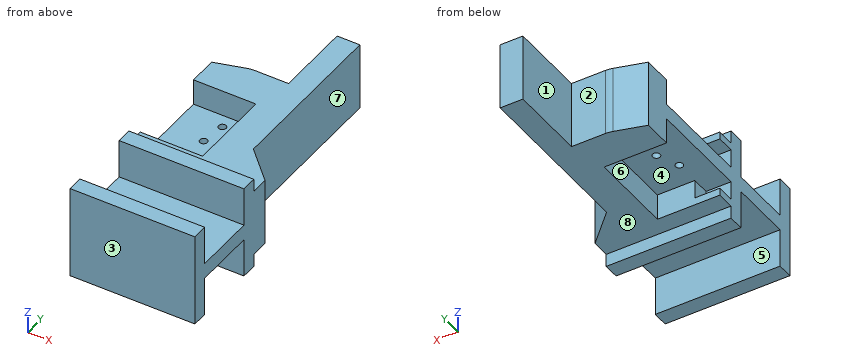
Autodesk Inventor part; units mm, degrees
ref_plane "YZ Plane" through (0, 0, 0) normal (1, 0, 0) x (0, 1, 0)
ref_plane "XZ Plane" through (0, 0, 0) normal (0, 1, 0) x (-1, 0, 0)
ref_plane "XY Plane" through (0, 0, 0) normal (0, 0, 1) x (1, 0, 0)
sketch "Sketch1" plane through (0, 0, 0) normal (0, 0, 1) x (1, 0, 0)
  line L0 (-9.525, 0) -> (9.525, 0)
  line L1 (9.525, 0) -> (9.525, 44.45)
  line L2 (9.525, 44.45) -> (5.715, 44.45)
  line L3 (5.715, 44.45) -> (4.891, 28.7274)
  line L4 (4.891, 28.7274) -> (-9.525, 28.7274)
  line L5 (-9.525, 28.7274) -> (-9.525, 0)
  point P0 (0, 0)
  point P1 (0, 0)
  dimension "d0" = 44.45
  dimension "d1" = 15.24
  dimension "d2" = 15.7226
  dimension "d3" = 19.05
  dimension "d14" = 93
extrude "Extrusion1" add sketch "Sketch1" along normal mid plane 15.7226
sketch "Sketch2" plane through (0, 0, 0) normal (1, 0, 0) x (0, 1, 0)
  line L0 (-19.05, 9.525) -> (-19.05, -9.525)
  line L1 (-19.05, -9.525) -> (-15.875, -9.525)
  line L2 (-15.875, -9.525) -> (-15.875, -1.5875)
  line L3 (-15.875, -1.5875) -> (-3.175, -1.5875)
  line L4 (-3.175, -1.5875) -> (-3.175, -9.525)
  line L5 (-3.175, -9.525) -> (0, -9.525)
  line L6 (0, -9.525) -> (0, 9.525)
  line L7 (0, 9.525) -> (-3.175, 9.525)
  line L8 (-3.175, 9.525) -> (-3.175, 1.5875)
  line L9 (-3.175, 1.5875) -> (-15.875, 1.5875)
  line L10 (-15.875, 1.5875) -> (-15.875, 9.525)
  line L11 (-15.875, 9.525) -> (-19.05, 9.525)
  line L12 (0, -7.8613) -> (0, 7.8613)
  point P0 (0, 0)
  point P1 (0, 0)
  dimension "d6" = 19.05
  dimension "d7" = 19.05
  dimension "d8" = 3.175
  dimension "d9" = 3.175
extrude "Extrusion2" add sketch "Sketch2" along normal mid plane 19.05
sketch "Sketch6" plane through (0, 0, 7.8613) normal (0, 0, 1) x (1, 0, 0)
  line L0 (4.891, 28.7274) -> (9.525, 28.7274)
  line L1 (9.525, 28.7274) -> (9.525, 44.45)
  line L2 (9.525, 44.45) -> (4.891, 44.45)
  line L3 (4.891, 44.45) -> (4.891, 28.7274)
  point P0 (0, 0)
extrude "Extrusion3" add sketch "Sketch6" against normal blind 15.7226
sketch "Sketch9" plane through (0, 0, 7.8613) normal (0, 0, 1) x (1, 0, 0)
  line L0 (4.891, 44.45) -> (4.891, 28.7274)
  line L1 (-9.525, 28.7274) -> (-9.525, 0)
  line L2 (4.891, 28.7274) -> (-2.729, 28.7274)
  line L3 (4.891, 28.7274) -> (-9.525, 28.7274)
  line L4 (-9.525, 28.7274) -> (-9.525, 26.7462)
  line L5 (-9.525, 26.7462) -> (-2.729, 28.7274)
  point P0 (0, 0)
  dimension "d22" = 14.416
  dimension "d23" = 7.62
  dimension "d24" = 1.9812
extrude "Extrusion5" cut sketch "Sketch9" against normal blind 25.4
fillet "Fillet2" radius 5.08 1 edges at (-2.729, 28.7274, 0)
sketch "Sketch10" plane through (-9.525, -15.875, 1.5875) normal (0, 0, 1) x (1, 0, 0)
  circle A0 centre (9.525, 6.35) radius 0.635
  line L0 (0, 0) -> (0, 12.7)
  line L1 (19.05, -3.175) -> (0, -3.175)
  point P0 (9.525, 15.875)
  dimension "d28" = 9.525
  dimension "d29" = 9.525
  dimension "d30" = 1.27
extrude "Extrusion6" cut sketch "Sketch10" against normal blind 25.4
sketch "Sketch12" plane through (-9.525, -15.875, -1.5875) normal (-1, 0, 0) x (0, 0, 1)
  line L0 (-6.2738, 60.325) -> (-6.2738, 15.875)
  line L1 (9.4488, 42.6212) -> (9.4488, 15.875)
  line L2 (-6.2738, 36.7601) -> (9.4488, 36.7601)
  line L3 (9.4488, 36.7601) -> (9.4488, 19.5053)
  line L4 (9.4488, 19.5053) -> (-6.2738, 19.5053)
  line L5 (-6.2738, 19.5053) -> (-6.2738, 36.7601)
  point P0 (1.5875, 15.875)
extrude "Extrusion7" cut sketch "Sketch12" against normal blind 12.7
sketch "Sketch13" plane through (3.175, -15.875, -1.5875) normal (-1, 0, 0) x (0, 0, 1)
  line L0 (0, 12.7) -> (0, 36.7601)
  line L1 (-6.2738, 36.7601) -> (9.4488, 36.7601)
  line L2 (0, 12.7) -> (0, 0)
  line L3 (3.175, 12.7) -> (3.175, 36.7601)
  line L4 (3.175, 0) -> (3.175, 12.7)
  line L5 (9.4488, 19.5053) -> (-6.2738, 19.5053)
  line L6 (0, 36.7601) -> (3.175, 36.7601)
  line L7 (3.175, 36.7601) -> (3.175, 19.5053)
  line L8 (3.175, 19.5053) -> (0, 19.5053)
  line L9 (0, 19.5053) -> (0, 36.7601)
  point P0 (1.5875, 15.875)
extrude "Extrusion8" add sketch "Sketch13" along normal blind 12.7
sketch "Sketch15" plane through (3.175, 3.6303, 1.5875) normal (0, 0, 1) x (1, 0, 0)
  circle A0 centre (-7.62, 5.0254) radius 0.635
  line L0 (-12.7, 0) -> (-12.7, 17.2548)
  circle A1 centre (-5.715, 9.4248) radius 0.635
  circle A2 centre (-5.08, 14.5048) radius 0.635
  point P0 (-3.175, -3.6303)
  dimension "d40" = 5.08
  dimension "d41" = 1.27
  dimension "d42" = 1.27
  dimension "d45" = 1.27
  dimension "d46" = 6.985
  dimension "d47" = 7.62
extrude "Extrusion9" cut sketch "Sketch15" against normal blind 12.7
sketch "Sketch17" plane through (-9.525, -15.875, -1.5875) normal (-1, 0, 0) x (0, 0, 1)
  line L0 (-7.9375, 15.875) -> (11.1125, 15.875)
  line L1 (0, 19.5053) -> (-3.81, 19.5053)
  line L2 (-3.81, 19.5053) -> (-3.81, 15.875)
  line L3 (-3.81, 15.875) -> (0, 15.875)
  line L4 (0, 15.875) -> (0, 19.5053)
  line L5 (3.175, 19.5053) -> (6.985, 19.5053)
  line L6 (6.985, 19.5053) -> (6.985, 15.875)
  line L7 (6.985, 15.875) -> (3.175, 15.875)
  line L8 (3.175, 15.875) -> (3.175, 19.5053)
  point P0 (1.5875, 15.875)
  dimension "d51" = 3.81
  dimension "d52" = 3.81
extrude "Extrusion10" cut sketch "Sketch17" against normal blind 5.08
sketch "Sketch18" plane through (9.525, 44.45, 7.8613) normal (1, 0, 0) x (0, 0, -1)
  line L0 (-1.6637, -63.5) -> (-1.6637, -60.325)
  line L1 (-1.6637, -60.325) -> (6.2738, -60.325)
  line L2 (6.2738, -60.325) -> (-1.6637, -60.325)
  line L3 (6.2738, -60.325) -> (6.2738, -47.625)
  line L4 (6.2738, -47.625) -> (-1.6637, -47.625)
  line L5 (-1.6637, -47.625) -> (-1.6637, -44.45)
  line L6 (-1.6637, -44.45) -> (-1.6637, -47.625)
  line L7 (-1.6637, -44.45) -> (0, -44.45)
  line L8 (0, -44.45) -> (0, -40.8197)
  line L9 (0, -44.45) -> (0, 0)
  line L10 (15.7226, 0) -> (15.7226, -44.45)
  line L11 (15.7226, -41.3057) -> (15.7226, -44.45)
  line L12 (17.3863, -44.45) -> (15.7226, -44.45)
  line L13 (15.7226, -44.45) -> (17.3863, -44.45)
  line L14 (17.3863, -44.45) -> (17.3863, -47.625)
  line L15 (17.3863, -47.625) -> (17.3863, -44.45)
  line L16 (17.3863, -47.625) -> (9.4488, -47.625)
  line L17 (9.4488, -47.625) -> (9.4488, -60.325)
  line L18 (17.3863, -60.325) -> (9.4488, -60.325)
  line L19 (9.4488, -60.325) -> (17.3863, -60.325)
  line L20 (17.3863, -63.5) -> (17.3863, -60.325)
  line L21 (17.3863, -60.325) -> (17.3863, -63.5)
  line L22 (17.3863, -63.5) -> (-1.6637, -63.5)
  line L23 (-1.6637, -63.5) -> (17.3863, -63.5)
  line L24 (0, -40.8197) -> (15.7226, -40.8197)
  line L25 (9.4488, -40.8197) -> (15.7226, -40.8197)
  line L26 (15.7226, -40.8197) -> (15.7226, -44.45)
  point P0 (7.8613, -44.45)
extrude "Extrusion11" add sketch "Sketch18" along normal blind 6.35
chamfer "Chamfer1" distance 6.35 angle 45 1 edges at (9.525, 3.6303, 0)
sketch "Sketch19" plane through (-9.525, -15.875, -1.5875) normal (0, 0, -1) x (-1, 0, 0)
  circle A0 centre (-9.525, 6.35) radius 0.762
  circle A1 centre (-9.525, 6.35) radius 0.635
  point P0 (-9.525, 15.875)
  dimension "d60" = 0
  dimension "d61" = 0
  dimension "d62" = 1.524
extrude "Extrusion12" cut sketch "Sketch19" against normal blind 6.35
sketch "Sketch20" plane through (3.175, 3.6303, -1.5875) normal (0, 0, -1) x (-1, 0, 0)
  circle A0 centre (5.08, 14.5048) radius 0.762
  circle A1 centre (5.08, 14.5048) radius 0.635
  circle A2 centre (5.715, 9.4248) radius 0.762
  circle A3 centre (5.715, 9.4248) radius 0.635
  circle A4 centre (7.62, 5.0254) radius 0.762
  circle A5 centre (7.62, 5.0254) radius 0.635
  point P0 (3.175, -3.6303)
  dimension "d65" = 0
  dimension "d66" = 0
  dimension "d67" = 1.524
  dimension "d68" = 0
  dimension "d69" = 0
  dimension "d70" = 1.524
  dimension "d71" = 0
  dimension "d72" = 0
  dimension "d73" = 1.524
extrude "Extrusion13" cut sketch "Sketch20" against normal blind 6.35
sketch "Sketch25" plane through (-9.525, -15.875, -1.5875) normal (-1, 0, 0) x (0, 0, 1)
  line L0 (9.4488, 19.5053) -> (9.4488, 15.875)
  line L1 (-6.2738, 15.875) -> (-6.2738, 19.5053)
  line L2 (-6.2738, 15.875) -> (-5.3086, 15.875)
  line L3 (-5.3086, 15.875) -> (-5.3086, 64.7795)
  line L4 (-5.3086, 64.7795) -> (-6.2738, 64.7795)
  line L5 (-6.2738, 64.7795) -> (-6.2738, 15.875)
  line L6 (9.4488, 15.875) -> (8.4836, 15.875)
  line L7 (8.4836, 15.875) -> (8.4836, 64.7795)
  line L8 (8.4836, 64.7795) -> (9.4488, 64.7795)
  line L9 (9.4488, 64.7795) -> (9.4488, 15.875)
  point P0 (1.5875, 15.875)
  dimension "d87" = 15.7226
  dimension "d88" = 0.9652
  dimension "d89" = 0.9652
extrude "Extrusion16" cut sketch "Sketch25" against normal blind 38.1
properties part number "mod_gripper" material "Steel, High Strength Low Alloy"
CAD build for the part. Positions are in the model's coordinates, mm. Face numbers are marked on the shaded views. A direction names the side the tool comes from. Coordinates: 2 decimals unless noted, no trailing zeros. Order: outer loops, then holes, each group sorted by start corner. A loop starts at its lowest first (then second) coordinate and runs counter-clockwise, first axis right, second up.
(1) Pin check, flat tips, straight feed: pin 1 Ø1.8 at (x, y) = (-7, 2) entering from -Z; pin 2 Ø7.5 at (x, z) = (0.5, -1.5) entering from +Y; pin 3 Ø1.9 at (x, z) = (-6.5, -3) entering from +Y (3 decimals); pin 4 Ø0.9 at (x, y) = (0, -9.525) entering from -Z. Stop position of each tip, or through.
Solution:
pin 1: stops at z = -6.9
pin 2: stops at y = 28.73
pin 3: stops at y = 27.905
pin 4: passes through
(2) Mould opens along Y. For the marked faces 1, 2, 3 and 4 say: released by +Y, released by -Y, zero draft, split by the parting line, or undercut.
Solution:
face 1: zero draft
face 2: released by +Y
face 3: released by -Y
face 4: undercut
(3) Which spindle directions (+Z, -Z, +X, -X, +Y, -Y) get a long thin tool onto all of the face, cutting with end or side? Do the marked faces 5, 6, 7 and 8. Say none if no direction does.
Solution:
face 5: -Z, +X, -X
face 6: -Z, -X
face 7: +Z, -Z, +X, +Y
face 8: -Z, +X, -X, +Y
(4) Drill centre lines: L1, parallel to Y at x = -1.5, z = 3.5 (3 decimals); L2, parallel to Y at x = 0, z = 0.9; L3, parallel to Y at x = -2, z = -7.75 (3 decimals). Where is each one in solid material? Low to high.
Solution:
L1: y = -19.05 to -15.875, -3.175 to 3.63, 20.885 to 28.727
L2: y = -19.05 to -10.29, -8.76 to 28.73
L3: y = -19.05 to -15.875, -3.175 to 0
(5) Saw through at C-C, the plane z = -8.5. Write the cut outline in (x, y) (3 decimals), and give its area (3 significant figures).
Solution:
outline: (-9.525, -19.05) - (15.875, -19.05) - (15.875, -15.875) - (-9.525, -15.875) - close; (-9.525, -3.175) - (15.875, -3.175) - (15.875, 0) - (-9.525, 0) - close
area: 161 mm2
